Design review of the part built by this model. Coordinates are the model's own, in mm. Face numbers are marked on the shaded views. A direction names the side the tool comes from. Give positions to 0.01 mm unless a question says otherwise; leave off trailing zeros. Loops run counter-clockwise (first coordinate to the right, second up) from the corner with the lowest first, then second, coordinate; pieces in that order, holes last.
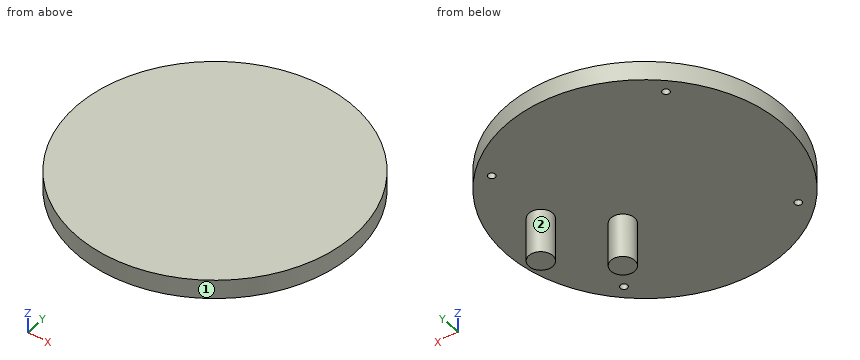
from build123d import *

# Parameters (mm, degrees)
CYLINDER_R      = 93.98
CYLINDER_DEPTH  = 12.954
SKETCH014_R     = 2.3876
POCKET006_DEPTH = 10.16
SKETCH015_R     = 8.001
PAD006_DEPTH    = 29.972


with BuildPart() as part:
    # Cylinder → Cylinder (new body)
    with BuildSketch(Plane(origin=(0, 0, -7.6454), x_dir=(1, 0, 0), z_dir=(0, 0, -1))):
        Circle(CYLINDER_R)
    extrude(amount=CYLINDER_DEPTH)

    # Sketch014 → Pocket006 (cut)
    with BuildSketch(Plane(origin=(0, 0, -20.5994), x_dir=(1, 0, 0), z_dir=(0, 0, -1))):
        with Locations((-59.718703, 59.718703)):
            Circle(SKETCH014_R)
        with Locations((59.718703, -59.718703)):
            Circle(SKETCH014_R)
        with Locations((59.718703, 59.718703)):
            Circle(SKETCH014_R)
        with Locations((-59.718703, -59.718703)):
            Circle(SKETCH014_R)
    extrude(amount=-POCKET006_DEPTH, mode=Mode.SUBTRACT)

    # Sketch015 → Pad006 (new body)
    with BuildSketch(Plane(origin=(0, 0, -20.5994), x_dir=(1, 0, 0), z_dir=(0, 0, -1))):
        with Locations((27.383657, 16.068535)):
            Circle(SKETCH015_R)
        with Locations((60.575206, -14.25543)):
            Circle(SKETCH015_R)
    extrude(amount=PAD006_DEPTH)


solid = part.part
Q1. Insertion check: pin 1 (5.5 mm diameter, centred on x = 60, y = -61, fed in from -Z); pin 2 (2.5 mm diameter, centred on x = 60, y = 60, fed in from -Z); pin 3 (2 mm diameter, centred on y = -8.5, z = -17.5, fed in from +X). Each pin has a flat end and moves straight along its axis. Give the tip position at first contact, or say it passes through.
Results:
pin 1: stops at z = -20.6
pin 2: stops at z = -10.44
pin 3: stops at x = 93.68
Q2. Take a section at B-B (z = -44.5). Give the boundary of the cut face in (x, y), plus the area to 3 significant figures.
Results:
outline: circle Ø16 at (27.38, -16.07); circle Ø16 at (60.58, 14.26)
area: 402 mm2
Q3. Wall thickness on line 1 (Z direction, x = -18.5, y = 19); line 2 (Y direction, x = 0.5, z = -19.5); line 3 (Y direction, x = -48, z = -12.5): over which ranges is each line inside the solid? List them lowest first.
Results:
line 1: z = -20.6 to -7.65
line 2: y = -93.98 to 93.98
line 3: y = -80.8 to 80.8
Q4. Tool access review of the marked faces 1 and 2: name each direction out of +Z, -Z, +X, -X, +Y, -Y from which nothing blocks a thin tool from reaching the whole face with its end or side.
Results:
face 1: +Z, -Z
face 2: -Z
Q5. Take a section at A-A (x = 0). Give the boundary of the cut face in (y, z).
Results:
outline: (-93.98, -20.6) - (93.98, -20.6) - (93.98, -7.65) - (-93.98, -7.65) - close
